from build123d import *

# Parameters (mm, degrees)
BOSS_EXTRU_1_DEPTH = 15
ESQUISSE2_W        = 10.1
ESQUISSE2_H        = 12
BOSS_EXTRU_2_DEPTH = 9
BOSS_EXTRU_3_DEPTH = 10
ESQUISSE4_R        = 2
BOSS_EXTRU_4_DEPTH = 1
BOSS_EXTRU_5_START = 1.6
ESQUISSE5_R        = 2
BOSS_EXTRU_5_DEPTH = 1.6
CONG_1_R           = 0.3


with BuildPart() as part:
    # Esquisse1 → Boss.-Extru.1 (new body)
    with BuildSketch(Plane.XY):
        with BuildLine():
            Line((5, -3.5), (5, 3.5))
            ThreePointArc((5, 3.5), (0, 6.05), (-5, 3.5))
            Line((-5, 3.5), (-5, -3.5))
            ThreePointArc((-5, -3.5), (0, -6.05), (5, -3.5))
        make_face()
    extrude(amount=BOSS_EXTRU_1_DEPTH)

    # Esquisse2 → Boss.-Extru.2 (add)
    with BuildSketch(Plane(origin=(0, 0, 0), x_dir=(-1, 0, 0), z_dir=(0, 0, -1))):
        Rectangle(ESQUISSE2_W, ESQUISSE2_H)
    extrude(amount=BOSS_EXTRU_2_DEPTH)

    # Esquisse3 → Boss.-Extru.3 (add)
    with BuildSketch(Plane(origin=(0, 0, -9), x_dir=(-1, 0, 0), z_dir=(0, 0, -1))):
        with BuildLine():
            Line((1, -1.118033989), (1, 1.118033989))
            ThreePointArc((1, 1.118033989), (-1.5, 0), (1, -1.118033989))
        make_face()
    extrude(amount=BOSS_EXTRU_3_DEPTH)

    # Esquisse4 → Boss.-Extru.4 (add)
    with BuildSketch(Plane(origin=(0, 0, -9), x_dir=(-1, 0, 0), z_dir=(0, 0, -1))):
        Circle(ESQUISSE4_R)
    extrude(amount=BOSS_EXTRU_4_DEPTH)

    # Esquisse5 → Boss.-Extru.5 (add)
    with BuildSketch(Plane.XY.offset(15).offset(BOSS_EXTRU_5_START)):
        with Locations(Location((0, 0, 0), (0, 0, 180))):
            Circle(ESQUISSE5_R)
    extrude(amount=-BOSS_EXTRU_5_DEPTH)

    # Congé1
    cong_1_edges = [part.edges().sort_by_distance(p)[0] for p in [
        (5.05, 6, -4.5),
        (5.05, -6, -4.5),
        (-5.05, -6, -4.5),
        (-5.05, 6, -4.5),
    ]]
    fillet(cong_1_edges, radius=CONG_1_R)


solid = part.part
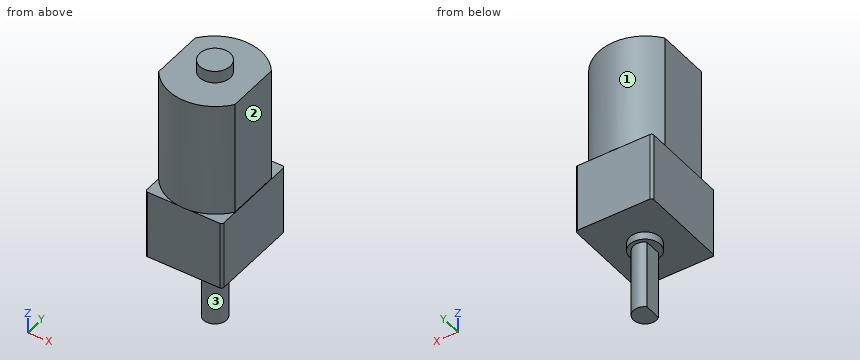
Could you check a few things on this model? Use its own coordinates, in mm. Face numbers are marked on the shaded views. A direction names the side the tool comes from. Coordinates: 2 decimals unless noted, no trailing zeros. Order: outer loops, then holes, each group sorted by start corner. A loop starts at its lowest first (then second) coordinate and runs counter-clockwise, first axis right, second up.
Q1. Will these pins go through, and if not, where does the flat tip stop? pin 1 (5 mm diameter, centred on y = 2, z = 9.5, fed in from +X); pin 2 (1.8 mm diameter, centred on y = 0, z = -15, fed in from -X); pin 3 (1.5 mm diameter, centred on x = -2.5, z = 9.5, fed in from -Y); pin 4 (1 mm diameter, centred on x = -2, z = -11, fed in from +Y).
Q2. Please list where these lines run through material, in increasing order: L1, parallel to Z at x = 3.75, y = 2; L2, parallel to Y at x = 4, z = -6.5; L3, parallel to X at y = -3.5, z = 9.
Q3. Suppose I cut it at D-D on y = 0. Please give me the cut outline in (x, z).
Q4. Suppose I cut it at C-C on z = 11. Please give me the cut outline in (x, y), and give its area (3 significant figures).
Q5. Suppose I cut it at B-B on y = -3. Please give me the cut outline in (x, z).
Q6. Which directions (+Z, -Z, +X, -X, +Y, -Y) give clear straight access to the entire face, cutting with the end or side of a thin tool? Please do the marked faces 1, 2 and 3.
Q7. Suppose I cut it at A-A on x = 0. Please give me the cut outline in (y, z), and give its area (3 significant figures).
Answer:
1. pin 1: stops at x = 5
1. pin 2: stops at x = -1
1. pin 3: stops at y = -5.8
1. pin 4: passes through
2. L1: z = -9 to 15
2. L2: y = -6 to 6
2. L3: x = -5 to 5
3. outline: (-5.05, -9) - (-2, -9) - (-2, -10) - (-1, -10) - (-1, -19) - (1.5, -19) - (1.5, -10) - (2, -10) - (2, -9) - (5.05, -9) - (5.05, 0) - (5, 0) - (5, 15) - (2, 15) - (2, 16.6) - (-2, 16.6) - (-2, 15) - (-5, 15) - (-5, 0) - (-5.05, 0) - close
4. outline: (-5, -3.5) arc R6.18 ccw to (5, -3.5) - (5, 3.5) arc R6.18 ccw to (-5, 3.5) - close
4. area: 106 mm2
5. outline: (-5.05, -9) - (5.05, -9) - (5.05, 0) - (5, 0) - (5, 15) - (-5, 15) - (-5, 0) - (-5.05, 0) - close
6. face 1: +Z, +Y
6. face 2: +Z, +X, +Y, -Y
6. face 3: -Z
7. outline: (-6.05, 0) - (-6, 0) - (-6, -9) - (-2, -9) - (-2, -10) - (-1.5, -10) - (-1.5, -19) - (1.5, -19) - (1.5, -10) - (2, -10) - (2, -9) - (6, -9) - (6, 0) - (6.05, 0) - (6.05, 15) - (2, 15) - (2, 16.6) - (-2, 16.6) - (-2, 15) - (-6.05, 15) - close
7. area: 327 mm2
